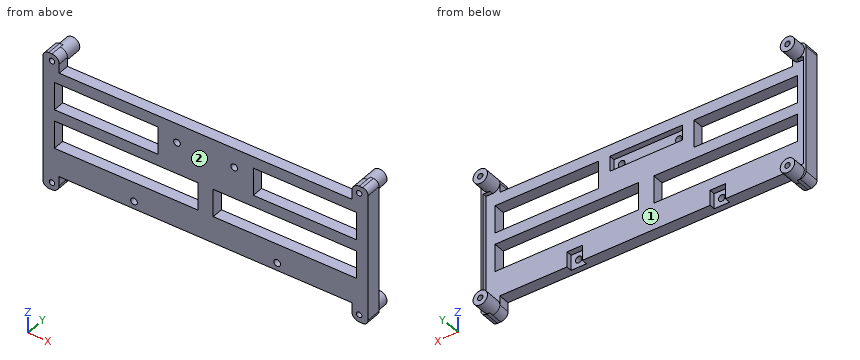
```python
from build123d import *

# Parameters (mm, degrees)
SCHIZZO1_R                   = 1.4
ESTRUSIONE_ESTRUSIONE1_DEPTH = 6
SCHIZZO2_R                   = 3.8
SCHIZZO2_R_2                 = 1.4
ESTRUSIONE_ESTRUSIONE2_DEPTH = 9
SCHIZZO3_R                   = 1.75
TAGLIO_ESTRUSIONE1_DEPTH     = 93.969080882
SCHIZZO5_W                   = 8
SCHIZZO5_H                   = 8
SCHIZZO5_W_2                 = 38
TAGLIO_ESTRUSIONE2_DEPTH     = 3
SCHIZZO6_W                   = 75.2
SCHIZZO6_H                   = 14.5
SCHIZZO6_W_2                 = 54.2
TAGLIO_ESTRUSIONE3_DEPTH     = 93.969080882
ESTRUSIONE_ESTRUSIONE4_DEPTH = 2
RACCORDO1_R                  = 3


with BuildPart() as part:
    # Schizzo1 → Estrusione-Estrusione1 (new body)
    with BuildSketch(Plane(origin=(0, 0, 0), x_dir=(1, 0, 0), z_dir=(0, 1, 0))):
        with BuildLine():
            Line((-76.7, -27.5), (-76.7, -32.3))
            ThreePointArc((-76.7, -32.3), (-77.812994231, -34.987005769), (-80.5, -36.1))
            Line((-80.5, -36.1), (-85.2, -36.1))
            Line((-85.2, -36.1), (-85.2, 36.1))
            Line((-85.2, 36.1), (-80.5, 36.1))
            ThreePointArc((-80.5, 36.1), (-77.812994231, 34.987005769), (-76.7, 32.3))
            Line((-76.7, 32.3), (-76.7, 27.5))
            Line((-76.7, 27.5), (76.7, 27.5))
            Line((76.7, 27.5), (76.7, 32.3))
            ThreePointArc((76.7, 32.3), (77.812994231, 34.987005769), (80.5, 36.1))
            Line((80.5, 36.1), (85.2, 36.1))
            Line((85.2, 36.1), (85.2, -36.1))
            Line((85.2, -36.1), (80.5, -36.1))
            ThreePointArc((80.5, -36.1), (77.812994231, -34.987005769), (76.7, -32.3))
            Line((76.7, -32.3), (76.7, -27.5))
            Line((76.7, -27.5), (-76.7, -27.5))
        make_face()
        with Locations(Location((-80.5, 32.3, 0), (0, 0, 270))):
            Circle(SCHIZZO1_R, mode=Mode.SUBTRACT)
        with Locations(Location((-80.5, -32.3, 0), (0, 0, 270))):
            Circle(SCHIZZO1_R, mode=Mode.SUBTRACT)
        with Locations(Location((80.5, -32.3, 0), (0, 0, 270))):
            Circle(SCHIZZO1_R, mode=Mode.SUBTRACT)
        with Locations(Location((80.5, 32.3, 0), (0, 0, 270))):
            Circle(SCHIZZO1_R, mode=Mode.SUBTRACT)
    extrude(amount=ESTRUSIONE_ESTRUSIONE1_DEPTH)

    # Schizzo2 → Estrusione-Estrusione2 (add)
    # profile 1 of 4: a face of its own
    with BuildSketch(Plane(origin=(0, 6, 0), x_dir=(1, 0, 0), z_dir=(0, 1, 0))):
        with Locations(Location((-80.5, 32.3, 0), (0, 0, 90))):
            Circle(SCHIZZO2_R)
        with Locations(Location((-80.5, 32.3, 0), (0, 0, 270))):
            Circle(SCHIZZO2_R_2, mode=Mode.SUBTRACT)
    # profile 2 of 4: a face of its own
    with BuildSketch(Plane(origin=(0, 6, 0), x_dir=(1, 0, 0), z_dir=(0, 1, 0))):
        with Locations(Location((-80.5, -32.3, 0), (0, 0, 270))):
            Circle(SCHIZZO2_R)
        with Locations(Location((-80.5, -32.3, 0), (0, 0, 270))):
            Circle(SCHIZZO2_R_2, mode=Mode.SUBTRACT)
    # profile 3 of 4: a face of its own
    with BuildSketch(Plane(origin=(0, 6, 0), x_dir=(1, 0, 0), z_dir=(0, 1, 0))):
        with Locations(Location((80.5, -32.3, 0), (0, 0, 270))):
            Circle(SCHIZZO2_R)
        with Locations(Location((80.5, -32.3, 0), (0, 0, 270))):
            Circle(SCHIZZO2_R_2, mode=Mode.SUBTRACT)
    # profile 4 of 4: a face of its own
    with BuildSketch(Plane(origin=(0, 6, 0), x_dir=(1, 0, 0), z_dir=(0, 1, 0))):
        with Locations(Location((80.5, 32.3, 0), (0, 0, 90))):
            Circle(SCHIZZO2_R)
        with Locations(Location((80.5, 32.3, 0), (0, 0, 270))):
            Circle(SCHIZZO2_R_2, mode=Mode.SUBTRACT)
    extrude(amount=ESTRUSIONE_ESTRUSIONE2_DEPTH)

    # Schizzo3 → Taglio-Estrusione1 (cut, through all)
    with BuildSketch(Plane(origin=(0, 6, 0), x_dir=(1, 0, 0), z_dir=(0, 1, 0))):
        with Locations(Location((-37.5, 23.5, 0), (0, 0, 270))):
            Circle(SCHIZZO3_R)
        with Locations(Location((-15, -17.5, 0), (0, 0, 270))):
            Circle(SCHIZZO3_R)
        with Locations(Location((15, -17.5, 0), (0, 0, 270))):
            Circle(SCHIZZO3_R)
        with Locations(Location((37.5, 23.5, 0), (0, 0, 270))):
            Circle(SCHIZZO3_R)
    extrude(amount=-TAGLIO_ESTRUSIONE1_DEPTH, mode=Mode.SUBTRACT)

    # Schizzo5 → Taglio-Estrusione2 (cut)
    with BuildSketch(Plane(origin=(0, 6, 0), x_dir=(1, 0, 0), z_dir=(0, 1, 0))):
        with Locations((37.5, 23.5)):
            Rectangle(SCHIZZO5_W, SCHIZZO5_H)
        with Locations((-37.5, 23.5)):
            Rectangle(SCHIZZO5_W, SCHIZZO5_H)
        with Locations((0, -17.5)):
            Rectangle(SCHIZZO5_W_2, SCHIZZO5_H)
    extrude(amount=-TAGLIO_ESTRUSIONE2_DEPTH, mode=Mode.SUBTRACT)

    # Schizzo6 → Taglio-Estrusione3 (cut, through all)
    with BuildSketch(Plane(origin=(0, 6, 0), x_dir=(1, 0, 0), z_dir=(0, 1, 0))):
        with Locations((-41.6, 6.25)):
            Rectangle(SCHIZZO6_W, SCHIZZO6_H)
        with Locations((41.6, 6.25)):
            Rectangle(SCHIZZO6_W, SCHIZZO6_H)
        with Locations((-52.1, -14.25)):
            Rectangle(SCHIZZO6_W_2, SCHIZZO6_H)
        with Locations((52.1, -14.25)):
            Rectangle(SCHIZZO6_W_2, SCHIZZO6_H)
    extrude(amount=-TAGLIO_ESTRUSIONE3_DEPTH, mode=Mode.SUBTRACT)

    # Schizzo7 → Estrusione-Estrusione4 (add)
    with BuildSketch(Plane(origin=(0, 6, 0), x_dir=(1, 0, 0), z_dir=(0, 1, 0))):
        with BuildLine():
            Line((-80.5, 36.1), (-85.2, 36.1))
            Line((-85.2, 36.1), (-85.2, -36.1))
            Line((-85.2, -36.1), (-80.5, -36.1))
            ThreePointArc((-80.5, -36.1), (-84.3, -32.3), (-80.5, -28.5))
            Line((-80.5, -28.5), (-84, -28.5))
            Line((-84, -28.5), (-84, 28.5))
            Line((-84, 28.5), (-80.5, 28.5))
            ThreePointArc((-80.5, 28.5), (-84.3, 32.3), (-80.5, 36.1))
        make_face()
    estrusione_estrusione4 = extrude(amount=ESTRUSIONE_ESTRUSIONE4_DEPTH)

    # Specchia3: Estrusione-Estrusione4 across plane
    add(estrusione_estrusione4.mirror(Plane(origin=(0, 0, 0), x_dir=(0, 0, 1), z_dir=(1, 0, 0))))

    # Raccordo1
    raccordo1_edges = [part.edges().sort_by_distance(p)[0] for p in [
        (85.2, 4, -36.1),
        (85.2, 4, 36.1),
        (-85.2, 3, 36.1),
        (-85.2, 3, -36.1),
    ]]
    fillet(raccordo1_edges, radius=RACCORDO1_R)


solid = part.part
```
Can you work these out from the model? Positions are in its coordinate system, mm. Face numbers are marked on the shaded views. Coordinates: 2 decimals unless noted, no trailing zeros. Loops run counter-clockwise (first coordinate to the right, second up) from the corner with the lowest first, then second, coordinate; pieces in that order, holes last. Notation, with made-up numbers: (-33, 46.25) - (-9, 46.25) arc R22 cw to (-9, 55.25) - close; hole circle Ø2 at (4, 18). An arc over 180 degrees is marked (long way). Answer as CSV lines item,"result". Start each with the question number.
1) For pin 1 (5 mm diameter, centred on x = -12.5, y = 6, fed in from -Z); pin 2 (5.5 mm diameter, centred on x = 15, z = 17.5, fed in from +Y); pin 3 (1 mm diameter, centred on x = -23.5, z = 21.5, fed in from -Y); pin 4 (1.7 mm diameter, centred on x = -80.5, z = 32.3, fed in from -Y), each with a flat end and sliding along its axis, tell me the tip position at first contact or that it passes through.
2) Suppose I cut it at D-D (z = -23.5). Please give me the cut outline in (x, y).
3) I need wall thicknesses on line 1 (X direction, y = 1.9, z = 17.5); line 2 (X direction, y = 2.15, z = -23.5); line 3 (Z direction, x = 80.5, y = 7). Which ranges of each line are inside material? Lowest first, please. Write a range as from..to.
4) Suppose I cut it at C-C (x = 37.5). Please give me the cut outline in (y, z).
5) Thinking about a two-plate mould opening in X: for the marked faces 1 and 2, which applies, pulls with the +X half, pulls with the -X half, needs draft (parallel to the pull), parting line crosses it, or undercut?
6) Suppose I cut it at A-A (y = 13). Please give me the cut outline in (x, z), plus the area to 3 significant figures.
7) Suppose I cut it at B-B (z = 17.5). Please give me the cut outline in (x, y), plus the area to 3 significant figures.
Check result:
1,pin 1,"stops at z = -27.5"
1,pin 2,"stops at y = 3"
1,pin 3,"stops at y = 0"
1,pin 4,"passes through"
2,outline,"(-85.2, 0) - (-39.25, 0) - (-39.25, 3) - (-41.5, 3) - (-41.5, 6) - (-84, 6) - (-84, 8) - (-85.2, 8) - close; (-35.75, 0) - (35.75, 0) - (35.75, 3) - (33.5, 3) - (33.5, 6) - (-33.5, 6) - (-33.5, 3) - (-35.75, 3) - close; (39.25, 0) - (85.2, 0) - (85.2, 8) - (84, 8) - (84, 6) - (41.5, 6) - (41.5, 3) - (39.25, 3) - close"
3,line 1,"x = -85.2..-79.2, -25..-16.75, -13.25..13.25, 16.75..25, 79.2..85.2"
3,line 2,"x = -85.2..-39.25, -35.75..35.75, 39.25..85.2"
3,line 3,"z = -36.1..-33.7, -30.9..-28.5, 28.5..30.9, 33.7..36.1"
4,outline,"(0, -27.5) - (3, -27.5) - (3, -25.25) - (0, -25.25) - close; (0, -21.75) - (3, -21.75) - (3, -19.5) - (6, -19.5) - (6, -13.5) - (0, -13.5) - close; (0, 1) - (6, 1) - (6, 7) - (0, 7) - close; (0, 21.5) - (6, 21.5) - (6, 27.5) - (0, 27.5) - close"
5,face 1,"undercut"
5,face 2,"needs draft"
6,outline,"circle Ø7.6 at (-80.5, -32.3); circle Ø7.6 at (-80.5, 32.3); circle Ø7.6 at (80.5, -32.3); circle Ø7.6 at (80.5, 32.3); hole circle Ø2.8 at (-80.5, -32.3); hole circle Ø2.8 at (-80.5, 32.3); hole circle Ø2.8 at (80.5, -32.3); hole circle Ø2.8 at (80.5, 32.3)"
6,area,"157 mm²"
7,outline,"(-85.2, 0) - (-79.2, 0) - (-79.2, 6) - (-84, 6) - (-84, 8) - (-85.2, 8) - close; (-25, 0) - (-16.75, 0) - (-16.75, 3) - (-19, 3) - (-19, 6) - (-25, 6) - close; (-13.25, 0) - (13.25, 0) - (13.25, 3) - (-13.25, 3) - close; (16.75, 0) - (25, 0) - (25, 6) - (19, 6) - (19, 3) - (16.75, 3) - close; (79.2, 0) - (85.2, 0) - (85.2, 8) - (84, 8) - (84, 6) - (79.2, 6) - close"
7,area,"242 mm²"
